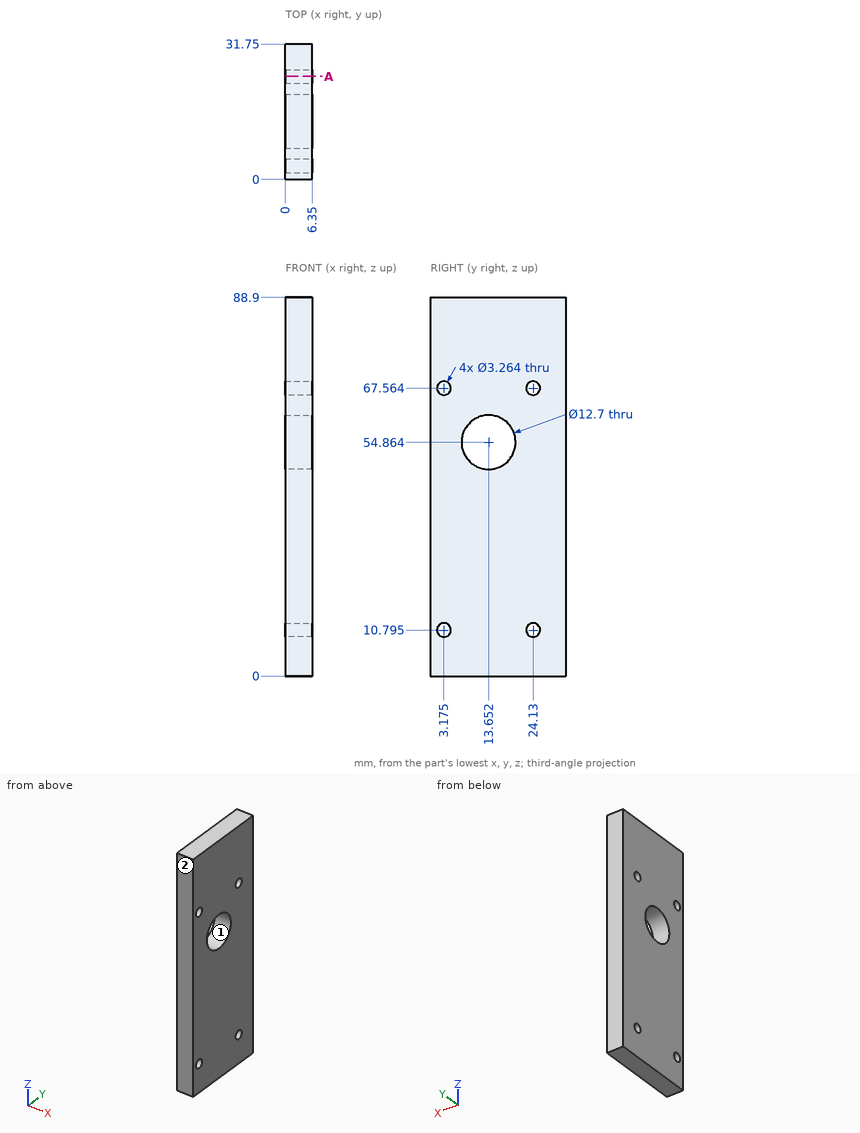
Verification items for this drawing (mm, ordinates from the low corner). Give positions to 0.01 mm unless a question says otherwise; leave off trailing zeros. Write item = value, one per line. Start each with the question number.
1. Go/stop test with flat-tipped pins: P1, Ø4, axis at y = 24.13, z = 10.795, coming from the -X side; P2, Ø11.5, axis at y = 13.65, z = 54.86, coming from the -X side. Record where each tip stops, or that it passes through.
2. Thickness scan on probe 1 along Z at (x, y) = (5.5, 24); probe 2 along Z at (x, y) = (2, 14) (1 decimal); probe 3 along Z at (x, y) = (4.75, 19) (1 decimal). Record the ranges inside material, lowest first.
3. Draft check along Z on the marked faces 1 and 2. Enter one of: +Z half, -Z half, draft (parallel to the pull), parting line (faces both ways), or undercut.
4. Section check A-A, the plane y = 24.13. Give the number of separate pieces and of enclosed holes in the cut face, plus the area to 3 significant figures.
Values follow:
q1.P1 = 0
q1.P2 = through
q2.probe_1 = 0 to 9.17, 12.42 to 65.94, 69.19 to 88.9
q2.probe_2 = 0 to 48.5, 61.2 to 88.9
q2.probe_3 = 0 to 51.4, 58.3 to 88.9
q3.face_1 = undercut
q3.face_2 = draft
q4.separate_pieces = 3
q4.enclosed_holes = 0
q4.area = 523 mm^2
